from build123d import *

# Parameters (mm, degrees)
PAD_DEPTH       = 13.1
POCKET_DEPTH    = 10.1
POCKET006_DEPTH = 6.1
SKETCH012_R     = 10
PAD003_DEPTH    = 7
SKETCH015_R     = 1
POCKET003_DEPTH = 6
POCKET004_DEPTH = 4.1
SKETCH013_R     = 3.75
POCKET001_DEPTH = 4
POCKET002_DEPTH = 1.6
SKETCH017_R     = 2
POCKET005_DEPTH = 5.5


with BuildPart() as part:
    # Sketch → Pad (new body)
    with BuildSketch(Plane.XY):
        with BuildLine():
            Line((-162, 6), (162, 6))
            ThreePointArc((166, 2), (164.828427, 4.828427), (162, 6))
            Line((166, 2), (166, -232))
            ThreePointArc((162, -236), (164.828427, -234.828427), (166, -232))
            Line((162, -236), (-162, -236))
            ThreePointArc((-166, -232), (-164.828427, -234.828427), (-162, -236))
            Line((-166, -232), (-166, 2))
            ThreePointArc((-162, 6), (-164.828427, 4.828427), (-166, 2))
        make_face()
    extrude(amount=PAD_DEPTH)

    # Sketch001 → Pocket (cut)
    with BuildSketch(Plane.XY.offset(13.1)):
        with BuildLine():
            Line((135, -8), (135, -142))
            ThreePointArc((132, -145), (134.12132, -144.12132), (135, -142))
            Line((132, -145), (-132, -145))
            ThreePointArc((-135, -142), (-134.12132, -144.12132), (-132, -145))
            Line((-135, -142), (-135, -8))
            ThreePointArc((-131.999986, -5), (-134.121315, -5.878675), (-135, -8))
            Line((-131.999986, -5), (-40.5, -5))
            ThreePointArc((-35, 0.5), (-38.889087, -1.110913), (-40.5, -5))
            Line((35, 0.5), (-35, 0.5))
            ThreePointArc((40.5, -5), (38.889087, -1.110913), (35, 0.5))
            Line((40.5, -5), (132, -5))
            ThreePointArc((135, -8), (134.12132, -5.87868), (132, -5))
        make_face()
    extrude(amount=-POCKET_DEPTH, mode=Mode.SUBTRACT)

    # Sketch018 → Pocket006 (cut)
    with BuildSketch(Plane.XY.offset(13.1)):
        with BuildLine():
            Line((-137.593576, 0.5), (138.406481, 0.5))
            ThreePointArc((141.406424, -2.518402), (140.534297, -0.385196), (138.406481, 0.5))
            Line((141.406424, -2.518402), (140.49521, -151.068141))
            ThreePointArc((137.495267, -154.049739), (139.610071, -153.177555), (140.49521, -151.068141))
            Line((137.495267, -154.049739), (-137.593576, -154.049739))
            ThreePointArc((-140.593576, -151.049739), (-139.714896, -153.171059), (-137.593576, -154.049739))
            Line((-140.593576, -151.049739), (-140.593576, -2.5))
            ThreePointArc((-137.593576, 0.5), (-139.714896, -0.37868), (-140.593576, -2.5))
        make_face()
    extrude(amount=-POCKET006_DEPTH, mode=Mode.SUBTRACT)

    # Sketch012 → Pad003 (join)
    with BuildSketch(Plane.XY):
        with Locations((-70, -120)):
            Circle(SKETCH012_R)
        with Locations((70, -120)):
            Circle(SKETCH012_R)
        with Locations((70, -30)):
            Circle(SKETCH012_R)
        with Locations((0, -90)):
            Circle(SKETCH012_R)
        with Locations((-70, -30)):
            Circle(SKETCH012_R)
    extrude(amount=PAD003_DEPTH)

    # Sketch015 → Pocket003 (cut)
    with BuildSketch(Plane.XZ.offset(-0.5)):
        with Locations((-11.3, 5.25)):
            Circle(SKETCH015_R)
        with BuildLine():
            ThreePointArc((2.75, 3), (5, 5.25), (2.75, 7.5))
            Line((2.75, 7.5), (-2.75, 7.5))
            ThreePointArc((-2.75, 7.5), (-5, 5.25), (-2.75, 3))
            Line((-2.75, 3), (2.75, 3))
        make_face()
    extrude(amount=-POCKET003_DEPTH, mode=Mode.SUBTRACT)

    # Sketch016 → Pocket004 (cut)
    with BuildSketch(Plane.XZ.offset(-1.9)):
        with BuildLine():
            Line((-4, 9.425651), (4, 9.425651))
            ThreePointArc((7, 6.425651), (6.12132, 8.546971), (4, 9.425651))
            Line((7, 6.425651), (7, 4.425651))
            ThreePointArc((4, 1.425651), (6.12132, 2.304331), (7, 4.425651))
            Line((4, 1.425651), (-4, 1.425651))
            ThreePointArc((-7, 4.425651), (-6.12132, 2.304331), (-4, 1.425651))
            Line((-7, 4.425651), (-7, 6.425651))
            ThreePointArc((-4, 9.425651), (-6.12132, 8.546971), (-7, 6.425651))
        make_face()
    extrude(amount=-POCKET004_DEPTH, mode=Mode.SUBTRACT)

    # Sketch013 → Pocket001 (cut)
    with BuildSketch(Plane.XY.offset(7)):
        with Locations((-70, -30)):
            Circle(SKETCH013_R)
        with Locations((-70, -120)):
            Circle(SKETCH013_R)
        with Locations((70, -120)):
            Circle(SKETCH013_R)
        with Locations((70, -30)):
            Circle(SKETCH013_R)
        with Locations((0, -90)):
            Circle(SKETCH013_R)
    extrude(amount=-POCKET001_DEPTH, mode=Mode.SUBTRACT)

    # Sketch014 → Pocket002 (cut)
    with BuildSketch(Plane.XY.offset(13.1)):
        with BuildLine():
            Line((-157, 0.5), (157, 0.5))
            ThreePointArc((161, -3.5), (159.828427, -0.671573), (157, 0.5))
            Line((161, -3.5), (161, -226.5))
            ThreePointArc((157, -230.5), (159.828427, -229.328427), (161, -226.5))
            Line((157, -230.5), (-157, -230.5))
            ThreePointArc((-161, -226.5), (-159.828427, -229.328427), (-157, -230.5))
            Line((-161, -226.5), (-161, -3.5))
            ThreePointArc((-157, 0.5), (-159.828427, -0.671573), (-161, -3.5))
        make_face()
    extrude(amount=-POCKET002_DEPTH, mode=Mode.SUBTRACT)

    # Sketch017 → Pocket005 (cut)
    with BuildSketch(Plane.XY.offset(11.5)):
        with Locations((-150, -10)):
            Circle(SKETCH017_R)
        with Locations((-150, -220)):
            Circle(SKETCH017_R)
        with Locations((150, -10)):
            Circle(SKETCH017_R)
        with Locations((150, -220)):
            Circle(SKETCH017_R)
    extrude(amount=-POCKET005_DEPTH, mode=Mode.SUBTRACT)


solid = part.part
Verification items for the finished model (mm, model axes). A direction names the side the tool comes from. Round coordinates to 2 decimals unless told otherwise and drop trailing zeros. Loops run counter-clockwise (first coordinate to the right, second up) from the corner with the lowest first, then second, coordinate; pieces in that order, holes last. Notation, with made-up numbers: (-16.75, 5) - (-2.75, 5) arc R17 cw to (-2.75, 36) - close; hole circle Ø4 at (65, 64.5). An arc over 180 degrees is marked (long way). Use a Markdown table: item, result. Add a question column.
1. Access from +Z, -Z, +X, -X, +Y, -Y to the whole of each face (thin tool, end or side, straight path). Record for faces 5 (the face through (0, 1.9, 8)), 6 (the face through (-2, -113, 0)), 7 (the face through (73.577, -118.874, 5.028)).
2. Section check A-A, the plane y = -170.5. Record the boundary of the cut face in (x, z), plus the area to 3 significant figures.
3. Gauge pin test, flat ends, axial feed: pin 1 (10 mm diameter, centred on x = -69.5, y = -124, fed in from +Z); pin 2 (10 mm diameter, centred on x = 98, y = -172, fed in from +Z); pin 3 (4 mm diameter, centred on x = 70, y = -119, fed in from +Z); pin 4 (4.5 mm diameter, centred on x = 70, y = -30, fed in from -Z). Record the tip position at first contact, or that the pin passes through.
4. Section check C-C, the plane y = -90. Record the boundary of the cut face in (x, z), plus the area to 3 significant figures.
5. Thickness scan on probe 1 along Y at (x, z) = (150, 9.7); probe 2 along Y at (x, z) = (0, 4.3); probe 3 along Y at (x, z) = (2, 8.25). Record the ranges inside material, lowest first. Write a range as [from, to].
6. Release check for a two-part mould opening along X. For faces 1 (the face through (-1.302, -80.085, 4.972)), 2 (the face through (-166, -117, 6)), 3 (the face through (-66.423, -28.874, 5.028)), 4 (the face through (2, -236, 6)) record: released by +X, released by -X, zero draft, split by the parting line, or undercut.
Checks:
| question | item | result |
|---|---|---|
| 1 | face 5 | +Y |
| 1 | face 6 | -Z, +X, -X, +Y, -Y |
| 1 | face 7 | +Z |
| 2 | outline | (-166, 0) - (166, 0) - (166, 13.1) - (161, 13.1) - (161, 11.5) - (-161, 11.5) - (-161, 13.1) - (-166, 13.1) - close |
| 2 | area | 3,830 mm^2 |
| 3 | pin 1 | stops at z = 7 |
| 3 | pin 2 | stops at z = 11.5 |
| 3 | pin 3 | stops at z = 3 |
| 3 | pin 4 | stops at z = 0 |
| 4 | outline | (-166, 0) - (166, 0) - (166, 13.1) - (161, 13.1) - (161, 11.5) - (140.87, 11.5) - (140.87, 7) - (135, 7) - (135, 3) - (10, 3) - (10, 7) - (3.75, 7) - (3.75, 3) - (-3.75, 3) - (-3.75, 7) - (-10, 7) - (-10, 3) - (-135, 3) - (-135, 7) - (-140.59, 7) - (-140.59, 11.5) - (-161, 11.5) - (-161, 13.1) - (-166, 13.1) - close |
| 4 | area | 1,540 mm^2 |
| 5 | probe 1 | y = [-236, -222], [-218, -12], [-8, 6] |
| 5 | probe 2 | y = [-236, -145], [-100, -93.75], [-86.25, -80] |
| 5 | probe 3 | y = [-236, -154.05], [0.5, 1.9] |
| 6 | face 1 | undercut |
| 6 | face 2 | released by -X |
| 6 | face 3 | undercut |
| 6 | face 4 | zero draft |
